from build123d import *

# Parameters (mm, degrees)
SKETCH1_W           = 70
SKETCH1_H           = 40
SKETCH1_R           = 1
BOSS_EXTRUDE1_DEPTH = 10


with BuildPart() as part:
    # Sketch1 → Boss-Extrude1 (new body)
    with BuildSketch(Plane.XY):
        Rectangle(SKETCH1_W, SKETCH1_H)
        with Locations((-14, 8)):
            Circle(SKETCH1_R, mode=Mode.SUBTRACT)
        with Locations(Location((14, 8, 0), (0, 0, 180))):
            Circle(SKETCH1_R, mode=Mode.SUBTRACT)
        with Locations((0, 8)):
            Circle(SKETCH1_R, mode=Mode.SUBTRACT)
        with Locations((-26.5, -10)):
            Circle(SKETCH1_R, mode=Mode.SUBTRACT)
        with Locations((-12.5, -10)):
            Circle(SKETCH1_R, mode=Mode.SUBTRACT)
        with Locations(Location((26.5, -10, 0), (0, 0, 180))):
            Circle(SKETCH1_R, mode=Mode.SUBTRACT)
        with Locations(Location((12.5, -10, 0), (0, 0, 180))):
            Circle(SKETCH1_R, mode=Mode.SUBTRACT)
    extrude(amount=BOSS_EXTRUDE1_DEPTH)


solid = part.part
Model file for the job. Use its own axes, mm. Give positions to 0.01 mm unless a question says otherwise; leave off trailing zeros. Loops run counter-clockwise (first coordinate to the right, second up) from the corner with the lowest first, then second, coordinate; pieces in that order, holes last.
1) Saw through at B-B (x = -26.5). Write the cut outline in (y, z).
2) Wall check: line 1 (Y direction, x = -26.5, z = 8); line 2 (Y direction, x = -14, z = 8.5). Give the ranges that are in metal, low to high.
3) Saw through at A-A (y = 8). Write the cut outline in (x, z), plus the area to 3 significant figures.
4) Pull direction Y, two halves, no side cores. Call faces 1 (the flat face through (0, 20, 5)), 2 (the flat face through (0, 0, 0)), 3 (the cylindrical face through (-13, 8, 5)): +Y half, -Y half, draft (parallel to the pull), parting line (faces both ways), or undercut.
5) Flat gauge pin, fed straight in: pin 1 Ø1.6 at (x, y) = (-14, 8) entering from -Z. Where does the tip first touch, or does it go through?
Answer block:
1. outline: (-20, 0) - (-11, 0) - (-11, 10) - (-20, 10) - close; (-9, 0) - (20, 0) - (20, 10) - (-9, 10) - close
2. line 1: y = -20 to -11, -9 to 20
2. line 2: y = -20 to 7, 9 to 20
3. outline: (-35, 0) - (-15, 0) - (-15, 10) - (-35, 10) - close; (-13, 0) - (-1, 0) - (-1, 10) - (-13, 10) - close; (1, 0) - (13, 0) - (13, 10) - (1, 10) - close; (15, 0) - (35, 0) - (35, 10) - (15, 10) - close
3. area: 640 mm2
4. face 1: +Y half
4. face 2: draft
4. face 3: undercut
5. pin 1: passes through
